CAD build for the part. Positions are in the model's coordinates, mm. Face numbers are marked on the shaded views. Round coordinates to 2 decimals unless told otherwise and drop trailing zeros. Loops run counter-clockwise (first coordinate to the right, second up) from the corner with the lowest first, then second, coordinate; pieces in that order, holes last. Notation, with made-up numbers: M 82,-11 L 104,-11 A14 ccw 104,11 Z; hole C 88.25,-15 d2. An arc over 180 degrees is marked long. Use a Markdown table: item, result. Add a question column.
(1) Flat gauge pins, fed straight in: P1, Ø4, axis at x = -0.5, y = -19, coming from the +Z side; P2, Ø4, axis at x = -8, y = -12.5, coming from the +Z side; P3, Ø3, axis at x = 0, z = -0.5, coming from the +Y side; P4, Ø4, axis at x = 3, y = -2.5, coming from the -Z side. Where does each tip first touch, or does it go through?
(2) Band-saw the part on D-D, the plane y = -15.75. Write the cut outline in (x, z), and give its area (3 significant figures).
(3) Band-saw the part on C-C, the plane x = 0. Write the cut outline in (y, z).
(4) Two-plate mould, pull along X, no slides. Class the marked faces 1, 2 and 3: released by +X, released by -X, zero draft, split by the parting line, or undercut.
(5) Band-saw the part on B-B, the plane y = -1.75. Write the cut outline in (x, z).
(6) Band-saw the part on A-A, the plane z = 0. Write the cut outline in (x, y).
(7) Wall check: L1, parallel to Z at x = 0, y = -8.25; L2, parallel to X at y = -20.25, z = 0.5; L3, parallel to X at y = -19, z = 4.5. Give the ranges that are in metal, low to high.
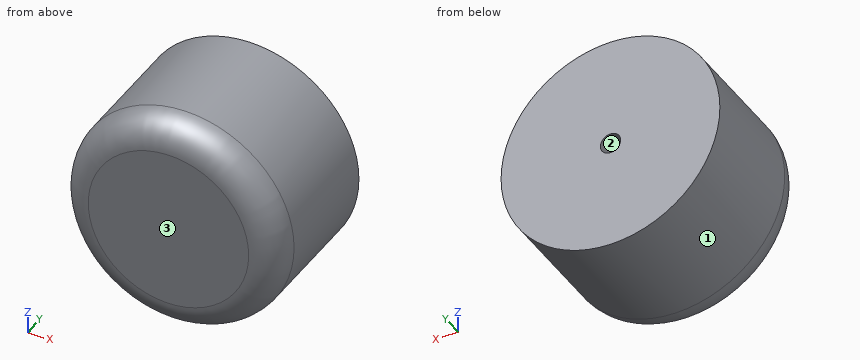
from build123d import *

# Parameters (mm, degrees)
F0_R     = 19.05
F1_DEPTH = 25.4
F2_R     = 21.73222
F2_R_2   = 19.05
F3_DEPTH = 19.05
F4_R     = 5.08
F5_R     = 1.761688
F6_DEPTH = 12.7


with BuildPart() as f1:
    # F0 (on Front) → F1 (new body)
    with BuildSketch(Plane.XZ):
        Circle(F0_R)
    extrude(amount=F1_DEPTH)

    # F2 (on face) → F3 (cut)
    with BuildSketch(Plane.XZ.offset(25.4)):
        Circle(F2_R)
        Circle(F2_R_2, mode=Mode.SUBTRACT)
    extrude(amount=-F3_DEPTH, mode=Mode.SUBTRACT)

    # F4
    f4_edges = [f1.edges().sort_by_distance(p)[0] for p in [
        (-19.05, -25.4, 0),
    ]]
    fillet(f4_edges, radius=F4_R)

    # F5 (on face) → F6 (cut)
    with BuildSketch(Plane(origin=(0, 0, 0), x_dir=(-1, 0, 0), z_dir=(0, 1, 0))):
        Circle(F5_R)
    extrude(amount=-F6_DEPTH, mode=Mode.SUBTRACT)


solid = f1.part
Return value:
| question | item | result |
|---|---|---|
| 1 | P1 | z = 19.05 |
| 1 | P2 | z = 18.08 |
| 1 | P3 | y = 0 |
| 1 | P4 | z = -19.02 |
| 2 | outline | C 0,0 d38.1 |
| 2 | area | 1,140 mm^2 |
| 3 | outline | M -25.4,-13.97 A5.08 ccw -20.32,-19.05 L 0,-19.05 L 0,-1.76 L -12.7,-1.76 L -12.7,1.76 L 0,1.76 L 0,19.05 L -20.32,19.05 A5.08 ccw -25.4,13.97 Z |
| 4 | face 1 | split by the parting line |
| 4 | face 2 | undercut |
| 4 | face 3 | zero draft |
| 5 | outline | C 0,0 d38.1; hole C 0,0 d3.52 |
| 6 | outline | M -19.05,-20.32 A5.08 ccw -13.97,-25.4 L 13.97,-25.4 A5.08 ccw 19.05,-20.32 L 19.05,0 L 1.76,0 L 1.76,-12.7 L -1.76,-12.7 L -1.76,0 L -19.05,0 Z |
| 7 | L1 | -19.05 to -1.76, 1.76 to 19.05 |
| 7 | L2 | -19.04 to 19.04 |
| 7 | L3 | -18.51 to 18.51 |
